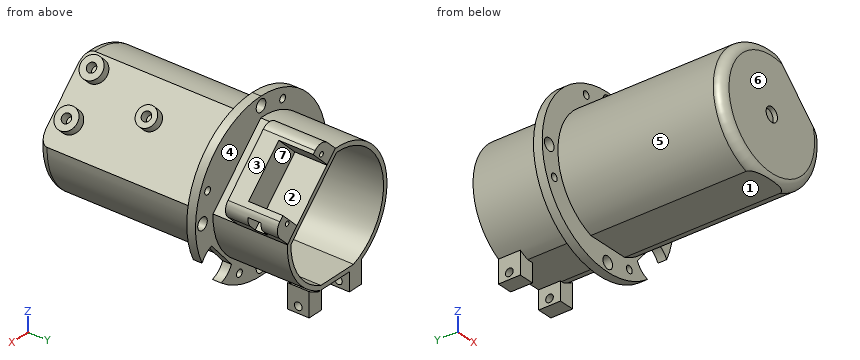
from build123d import *

# Parameters (mm, degrees)
SKETCH1_R            = 37.500000000000014
BOSS_EXTRUDE1_DEPTH  = 4
BOSS_EXTRUDE2_DEPTH  = 34
SKETCH5_R            = 2.7499999996325837
SKETCH5_R_2          = 2.75
SKETCH5_R_3          = 2.7500000000258247
SKETCH5_R_4          = 2.749999999658416
SKETCH5_R_5          = 1.6500000000000001
SKETCH5_R_6          = 1.6499999999999988
SKETCH5_R_7          = 1.6499999999999957
CUT_EXTRUDE2_DEPTH   = 10
BOSS_EXTRUDE6_DEPTH  = 75
SHELL1_T             = -2
CUT_EXTRUDE3_DEPTH   = 10
FILLET1_R            = 4
BOSS_EXTRUDE9_DEPTH  = 10
SKETCH21_R           = 1.7500000000000104
CUT_EXTRUDE5_DEPTH   = 40
BOSS_EXTRUDE13_DEPTH = 12.999999999999998
FILLET2_R            = 5
SKETCH28_R           = 1.05
SKETCH28_R_2         = 1.049999999999999
CUT_EXTRUDE11_DEPTH  = 5.999999999999993
SKETCH29_R           = 3.25
CUT_EXTRUDE12_DEPTH  = 5.999999999999993
SKETCH31_W           = 8
SKETCH31_H           = 5.999999999999993
CUT_EXTRUDE13_DEPTH  = 10
BOSS_EXTRUDE14_START = -28
BOSS_EXTRUDE14_DEPTH = 10
SKETCH33_R           = 4.9999999999920695
SKETCH33_R_2         = 4.499999999992068
BOSS_EXTRUDE15_DEPTH = 3.86
SKETCH34_R           = 2.0999999999920713
SKETCH34_R_2         = 2.099999999992072
SKETCH34_R_3         = 2.0999999999920704
CUT_EXTRUDE14_DEPTH  = 4.2
CUT_EXTRUDE15_DEPTH  = 6
CUT_EXTRUDE16_DEPTH  = 1.082123817


with BuildPart() as part:
    # Sketch1 → Boss-Extrude1 (new body)
    with BuildSketch(Plane(origin=(0, 0, 0), x_dir=(1, 0, 0), z_dir=(0, 1, 0))):
        with Locations(Location((0, 0, 0), (0, 0, 270))):
            Circle(SKETCH1_R)
    extrude(amount=BOSS_EXTRUDE1_DEPTH)

    # Sketch3 → Boss-Extrude2 (add)
    with BuildSketch(Plane(origin=(0, 4, 0), x_dir=(1, 0, 0), z_dir=(0, 1, 0))):
        with BuildLine():
            Line((27.43260268125508, -1.224872854444847), (0.18369490524426094, -28.473671452031667))
            ThreePointArc((0.18369490524426094, -28.473671452031667), (-29.000581799821436, -5.524070669091407), (-10.736939275039097, 26.800000000011135))
            Line((-10.736939275039097, 26.800000000011135), (8.654811548442561, 26.800000000011135))
            ThreePointArc((8.654811548442561, 26.800000000011135), (22.63544047994107, 15.864209469271458), (27.43260268125508, -1.224872854444847))
        make_face()
        with BuildLine():
            Line((25.45631471019754, -0.37273144868234936), (-0.6684385820861921, -26.49738006670114))
            ThreePointArc((-0.6684385820861921, -26.49738006670114), (-27.07858694278502, -4.929238469082694), (-10.379693313062322, 24.80000000001113))
            Line((-10.379693313062322, 24.80000000001113), (8.297565586465787, 24.80000000001113))
            ThreePointArc((8.297565586465787, 24.80000000001113), (20.85577312079139, 14.925767320058823), (25.45631471019754, -0.37273144868234936))
        make_face(mode=Mode.SUBTRACT)
    extrude(amount=BOSS_EXTRUDE2_DEPTH)

    # Sketch5 → Cut-Extrude2 (cut)
    with BuildSketch(Plane(origin=(0, 4, 0), x_dir=(1, 0, 0), z_dir=(0, 1, 0))):
        with Locations(Location((-33.49492446290215, 0.00013411391513071, 0), (0, 0, 270))):
            Circle(SKETCH5_R)
        with Locations(Location((-0.00013356723643175, 33.494790805725295, 0), (0, 0, 270))):
            Circle(SKETCH5_R_2)
        with Locations(Location((33.494523124573746, -8.994042047e-08, 0), (0, 0, 270))):
            Circle(SKETCH5_R_3)
        with Locations(Location((-0.00026777109197641, -33.49465678175059, 0), (0, 0, 270))):
            Circle(SKETCH5_R_4)
        with Locations(Location((-12.362017582725011, -30.59706720070402, 0), (0, 0, 270))):
            Circle(SKETCH5_R_5)
        with Locations(Location((-30.59706720070398, 12.362017582725123, 0), (0, 0, 270))):
            Circle(SKETCH5_R_6)
        with Locations(Location((12.362017582725228, 30.59706720070393, 0), (0, 0, 270))):
            Circle(SKETCH5_R_5)
        with Locations(Location((30.597067200703897, -12.362017582725326, 0), (0, 0, 270))):
            Circle(SKETCH5_R_7)
    extrude(amount=-CUT_EXTRUDE2_DEPTH, mode=Mode.SUBTRACT)

    # Sketch16 → Cut-Extrude3 (cut)
    with BuildSketch(Plane(origin=(0, 4, 0), x_dir=(1, 0, 0), z_dir=(0, 1, 0))):
        with BuildLine():
            Line((0.3726252811901698, -26.49738006670113), (26.4973785734739, -0.3727314486823372))
            ThreePointArc((26.4973785734739, -0.3727314486823372), (-18.738292161801, 18.738367240979606), (0.3726252811901698, -26.49738006670113))
        make_face()
    extrude(amount=-CUT_EXTRUDE3_DEPTH, mode=Mode.SUBTRACT)

    # Sketch18 → Boss-Extrude9 (add)
    with BuildSketch(Plane(origin=(0, 38.00000000000001, 0), x_dir=(1, 0, 0), z_dir=(0, 1, 0))):
        with BuildLine():
            Line((15, 24.233241632102853), (14.999999999999998, 35.23324163210285))
            Line((14.999999999999998, 35.23324163210285), (7.9999999999999964, 35.23324163210285))
            Line((7.9999999999999964, 35.23324163210285), (7.999999999999998, 26.80000000001115))
            Line((7.999999999999998, 26.80000000001115), (9.695875411718896, 26.80000000001115))
            ThreePointArc((9.695875411718896, 26.80000000001115), (12.414452372843087, 25.654071261350285), (15, 24.233241632102853))
        make_face()
        with BuildLine():
            Line((-7.9999999999999964, 35.23324163210285), (-7.999999999999998, 26.800000000011156))
            Line((-7.999999999999998, 26.800000000011156), (-9.695875411762707, 26.800000000011156))
            ThreePointArc((-9.695875411762707, 26.800000000011156), (-12.414452372860087, 25.65407126133764), (-15, 24.233241632102853))
            Line((-15, 24.233241632102853), (-14.999999999999998, 35.23324163210285))
            Line((-14.999999999999998, 35.23324163210285), (-7.9999999999999964, 35.23324163210285))
        make_face()
    extrude(amount=-BOSS_EXTRUDE9_DEPTH)

    # Sketch21 → Cut-Extrude5 (cut)
    with BuildSketch(Plane(origin=(15.000000000000004, 0, -2.37e-15), x_dir=(1.6e-16, 0, -1), z_dir=(1, 0, 1.6e-16))):
        with Locations((32.233241632105404, 33.000000000000185)):
            Circle(SKETCH21_R)
    extrude(amount=-CUT_EXTRUDE5_DEPTH, mode=Mode.SUBTRACT)

    # Sketch27 → Boss-Extrude13 (add)
    with BuildSketch(Plane(origin=(14.328682810517009, 0, 14.328740221598881), x_dir=(0.7071081977732587, 0, -0.7071053645969985), z_dir=(0.7071053645969985, 0, 0.7071081977732587))):
        Polygon((-13.356558336469002, 23.382123816577263), (-13.356558336469002, 39.082123816577024), (-19.94256467636435, 39.082123816577024), (-19.94256467636435, 15.382123816577272), (18.593133059597207, 15.382123816577272), (18.5931330595972, 39.082123816577024), (11.123133059597205, 39.082123816577024), (11.123133059597208, 23.382123816577263), align=None)
    extrude(amount=BOSS_EXTRUDE13_DEPTH)

    # Fillet2
    fillet2_edges = [part.edges().sort_by_distance(p)[0] for p in [
        (36.66840935900816, 27.23212381657715, 10.373842661544257),
        (9.419501582997341, 27.232123816577147, 37.62264125913108),
    ]]
    fillet(fillet2_edges, radius=FILLET2_R)

    # Sketch28 → Cut-Extrude11 (cut)
    with BuildSketch(Plane(origin=(0, 39.082123816577024, 0), x_dir=(1, 0, 0), z_dir=(0, 1, 0))):
        with Locations(Location((9.316450186911645, -30.79605966921365, 0), (0, 0, 270))):
            Circle(SKETCH28_R)
        with Locations(Location((28.97405808500825, -11.138530533417102, 0), (0, 0, 270))):
            Circle(SKETCH28_R_2)
    extrude(amount=-CUT_EXTRUDE11_DEPTH, mode=Mode.SUBTRACT)

    # Sketch31 → Cut-Extrude13 (cut)
    with BuildSketch(Plane(origin=(13.14735680873018, 4.81e-15, -13.147304131106994), x_dir=(-0.7071053645969986, 0, -0.7071081977732586), z_dir=(0.7071081977732586, 0, -0.7071053645969986))):
        with Locations((-28.36385815738135, 28.661507762433622)):
            Rectangle(SKETCH31_W, SKETCH31_H)
    extrude(amount=-CUT_EXTRUDE13_DEPTH, mode=Mode.SUBTRACT)



with BuildPart() as body_2:
    # Sketch15 → Boss-Extrude6 (new body)
    with BuildSketch(Plane.XZ):
        with BuildLine():
            Line((28.473666544542198, 1.2248728544340861), (1.2247587685206183, 28.47367145203166))
            ThreePointArc((1.2247587685206183, 28.47367145203166), (-27.95951793651176, 5.524070669097932), (-9.695875411762707, -26.800000000011156))
            Line((-9.695875411762707, -26.800000000011156), (9.695875411718896, -26.80000000001115))
            ThreePointArc((9.695875411718896, -26.80000000001115), (23.676504343229105, -15.864209469281034), (28.473666544542198, 1.2248728544340861))
        make_face()
    extrude(amount=BOSS_EXTRUDE6_DEPTH)

    # Shell1
    shell1_openings = [body_2.faces().sort_by_distance(p)[0] for p in [
        (-1.446451, 0, -1.185792841),
    ]]
    offset(amount=SHELL1_T, openings=shell1_openings, kind=Kind.INTERSECTION)

    # Fillet1
    fillet1_edges = [body_2.edges().sort_by_distance(p)[0] for p in [
        (-27.95951793651426, -75, 5.524070669085284),
    ]]
    fillet(fillet1_edges, radius=FILLET1_R - 0.0001)  # a hair under: the kernel refuses the full size

    # Sketch29 → Cut-Extrude12 (cut)
    with BuildSketch(Plane(origin=(0, -73, 0), x_dir=(1, 0, 0), z_dir=(0, 1, 0))):
        with Locations(Location((0, 0, 0), (0, 0, 270))):
            Circle(SKETCH29_R)
    extrude(amount=-CUT_EXTRUDE12_DEPTH, mode=Mode.SUBTRACT)


with BuildPart() as part_1:
    add(part.part)

    add(body_2.part)  # Boss-Extrude14 merges body 2
    # Sketch32 → Boss-Extrude14 (add)
    with BuildSketch(Plane(origin=(0, 38.00000000000001, 0), x_dir=(1, 0, 0), z_dir=(0, 1, 0)).offset(BOSS_EXTRUDE14_START)):
        with BuildLine():
            Line((-9.338629449742895, 24.800000000011153), (9.338629449721768, 24.800000000011146))
            ThreePointArc((9.338629449721768, 24.800000000011146), (-9.8838e-12, 26.499999999995538), (-9.338629449742895, 24.800000000011153))
        make_face()
    extrude(amount=-BOSS_EXTRUDE14_DEPTH)

    # Sketch33 → Boss-Extrude15 (add)
    with BuildSketch(Plane(origin=(14.849212656531403, 0, 14.849272153232874), x_dir=(0.7071081977732585, 0, -0.7071053645969986), z_dir=(0.7071053645969986, 0, 0.7071081977732585))):
        with Locations(Location((-12.878558963055134, -66.6999115263342, 0), (0, 0, 180))):
            Circle(SKETCH33_R)
        with Locations(Location((7.461441036944884, -66.6999115263342, 0), (0, 0, 180))):
            Circle(SKETCH33_R)
        with Locations(Location((-4.153697003459532, -36.6999367707353, 0), (0, 0, 180))):
            Circle(SKETCH33_R_2)
    extrude(amount=BOSS_EXTRUDE15_DEPTH)

    # Sketch34 → Cut-Extrude14 (cut)
    with BuildSketch(Plane(origin=(17.578639363876515, -2.8e-15, 17.578709796638343), x_dir=(0.7071081977732586, 0, -0.7071053645969986), z_dir=(0.7071053645969986, 0, 0.7071081977732586))):
        with Locations((-4.153697003459547, -36.69993677073529)):
            Circle(SKETCH34_R)
        with Locations((7.46144103694487, -66.6999115263342)):
            Circle(SKETCH34_R_2)
        with Locations((-12.87855896305515, -66.69991152633419)):
            Circle(SKETCH34_R_3)
    extrude(amount=-CUT_EXTRUDE14_DEPTH, mode=Mode.SUBTRACT)

    # Sketch35 → Cut-Extrude15 (cut)
    with BuildSketch(Plane(origin=(0, 4, 0), x_dir=(1, 0, 0), z_dir=(0, 1, 0))):
        with BuildLine():
            Line((16.930501479421057, 24.731996700817078), (28.25712370299877, 11.758011181218741))
            ThreePointArc((28.25712370299877, 11.758011181218741), (32.49604489503215, 26.889906797281803), (16.930501479421057, 24.731996700817078))
        make_face()
    extrude(amount=-CUT_EXTRUDE15_DEPTH, mode=Mode.SUBTRACT)

    # Sketch36 → Cut-Extrude16 (cut)
    with BuildSketch(Plane(origin=(0, 39.082123816577024, 0), x_dir=(1, 0, 0), z_dir=(0, 1, 0))):
        Polygon((27.47603961924718, -1.181436090491898), (28.646536061254768, -2.3519372223451054), (1.397628285210752, -29.600735819898734), (0.22713184323636287, -28.430234688078716), align=None)
    extrude(amount=-CUT_EXTRUDE16_DEPTH, mode=Mode.SUBTRACT)


solid = part_1.part
The listing builds one solid part. Answer for the finished solid, in the listing's coordinates (mm). Face numbers are marked on the shaded views. A direction names the side the tool comes from. Coordinates: 2 decimals unless noted, no trailing zeros. Loops run counter-clockwise (first coordinate to the right, second up) from the corner with the lowest first, then second, coordinate; pieces in that order, holes last.
1) Determine the mould class of the marked faces 4, 5, 6 and 7 for opening direction Y: pulls with the +Y half, pulls with the -Y half, needs draft (parallel to the pull), parting line crosses it, or undercut.
2) Flat-ended cylindrical pins translate along their axes: pin 1 Ø5 at (x, z) = (0, 0) entering from +Y; pin 2 Ø3.5 at (x, z) = (28.97, 11.14) entering from -Y; pin 3 Ø10 at (y, z) = (4.5, -4) entering from -X; pin 4 Ø8 at (x, z) = (-9.5, 26.5) entering from -Y. Find the tip coordinate at first contact, or state that the pin passes through.
3) Find section A-A on y = -19.5. Write down the section's boundary in (x, z).
4) Find the intervals of material crossed by L1, parallel to X at y = 1.25, z = 0; L2, parallel to Y at x = 27.5, z = 7; L3, parallel to Y at x = 10, z = 34, in increasing order.
5) A tool of negligible diameter and unlimited length cuts with its end or side. For the marked faces 1, 2 and 3, from which of +Z, -Z, +X, -X, +Y, -Y can it reach the whole face along a straight path? Write none if from no direction.
Values:
1. face 4: undercut
1. face 5: needs draft
1. face 6: pulls with the -Y half
1. face 7: pulls with the +Y half
2. pin 1: passes through
2. pin 2: stops at y = 0
2. pin 3: stops at x = -37.5
2. pin 4: stops at y = -75
3. outline: (-9.7, -26.8) - (9.7, -26.8) arc R28.5 ccw to (28.47, 1.22) - (1.22, 28.47) arc R28.5 ccw to start; hole (-9.34, -24.8) - (9.34, -24.8) arc R26.5 ccw to (26.5, 0.37) - (0.37, 26.5) arc R26.5 ccw to start
4. L1: x = -37.5 to -36.24, -30.74 to -26.5, 26.5 to 30.74, 36.24 to 37.5
4. L2: y = 0 to 4, 15.38 to 25.66, 31.66 to 39.08
4. L3: y = 0 to 4, 15.38 to 39.08
5. face 1: -Z, +X, -X, -Y
5. face 2: +Y
5. face 3: +Z, +X, +Y
